Here's how the part is built. I have some questions about the finished solid (model axes, mm). A direction names the side the tool comes from. Round coordinates to 2 decimals unless told otherwise and drop trailing zeros. Write each loop counter-clockwise with the first axis right and the second up, starting at its lowest first coordinate (ties: lowest second). Pieces come first, ordered by that corner, then holes. Notation, with made-up numbers: (88, 68) - (132, 68) arc R16 cw to (132, 87) - close; hole circle Ø3 at (44, 27.5). An arc over 180 degrees is marked (long way). Use one line per item in the form item = value. Start each with the question number.
1. I want a section at A-A, the plane x = -13. List the corners of the cut face in (y, z) for me (3 decimals), plus the area to 3 significant figures.
2. Which directions (+Z, -Z, +X, -X, +Y, -Y) give clear straight access to the entire face, cutting with the end or side of a thin tool? Please do faces 1 (the flat face through (-21, 5, 17.805)), 2 (the flat face through (-99, 5, 14.805)), 3 (the flat face through (-86, 5, -86.155)).
3. I want a section at B-B, the plane y = 7. List the corners of the cut face in (x, z) for me (3 decimals), plus the area to 3 significant figures.
4. If I drill on line 1 along Z through (x, y) = (-58.5, 1) (3 decimals); line 2 along Z through (x, y) = (-132, 3.5) (3 decimals), over which ranges is the centre line in solid material (lowest first)?
5. Will these pins go through, and if not, where does the flat tip stop? pin 1 (2 mm diameter, centred on x = -5.5, y = 4, fed in from +Z) (3 decimals); pin 2 (1.8 mm diameter, centred on x = -52.5, y = 1, fed in from -Z) (3 decimals); pin 3 (3.5 mm diameter, centred on x = -6.49, z = 23.8, fed in from +Y); pin 4 (2.5 mm diameter, centred on x = -163.39, z = -91.16, fed in from -Y).
```python
from build123d import *

# Parameters (mm, degrees)
SKETCH1_R           = 1.5
BOSS_EXTRUDE1_DEPTH = 1.6
BOSS_EXTRUDE2_DEPTH = 7


with BuildPart() as part:
    # Sketch1 → Boss-Extrude1 (new body)
    with BuildSketch(Plane(origin=(0, 0, 0), x_dir=(1, 0, 0), z_dir=(0, 1, 0))):
        Polygon((-167.387715517, 87.155002586), (-167.387715517, -19.804997414), (-167.387715517, -28.459997414), (-159.387715517, -28.459997414), (-159.387715517, -19.804997414), (-10.487715517, -19.804997414), (-10.487715517, -28.459997414), (-2.487715517, -28.459997414), (-2.487715517, -19.804997414), (-2.487715517, 87.155002586), (-2.487715517, 95.810002586), (-10.487715517, 95.810002586), (-10.487715517, 87.155002586), (-159.387715517, 87.155002586), (-159.387715517, 95.810002586), (-167.387715517, 95.810002586), align=None)
        with Locations(Location((-6.487715517, -23.804997414, 0), (0, 0, 270))):
            Circle(SKETCH1_R, mode=Mode.SUBTRACT)
        with Locations(Location((-163.387715517, -23.804997414, 0), (0, 0, 270))):
            Circle(SKETCH1_R, mode=Mode.SUBTRACT)
        with Locations(Location((-6.487715517, 91.155002586, 0), (0, 0, 90))):
            Circle(SKETCH1_R, mode=Mode.SUBTRACT)
        with Locations(Location((-163.387715517, 91.155002586, 0), (0, 0, 90))):
            Circle(SKETCH1_R, mode=Mode.SUBTRACT)
    extrude(amount=BOSS_EXTRUDE1_DEPTH)

    # Sketch2 → Boss-Extrude2 (add)
    with BuildSketch(Plane(origin=(0, 1.6, 0), x_dir=(1, 0, 0), z_dir=(0, 1, 0))):
        Polygon((-167.387715517, 86.155002586), (-2.487715517, 86.155002586), (-2.487715517, -14.804997414), (-10.487715517, -14.804997414), (-10.487715517, -17.804997414), (-32.487715517, -17.804997414), (-32.487715517, -14.804997414), (-167.387715517, -14.804997414), align=None)
    extrude(amount=BOSS_EXTRUDE2_DEPTH)


solid = part.part
```
Model answer:
q1.outline = (0, -87.155) - (1.6, -87.155) - (1.6, -86.155) - (8.6, -86.155) - (8.6, 17.805) - (1.6, 17.805) - (1.6, 19.805) - (0, 19.805) - close
q1.area = 899 mm2
q2.face_1 = +Z, +X, -X, +Y
q2.face_2 = +Z, -X, +Y
q2.face_3 = -Z, +X, -X, +Y
q3.outline = (-167.388, -86.155) - (-2.488, -86.155) - (-2.488, 14.805) - (-10.488, 14.805) - (-10.488, 17.805) - (-32.488, 17.805) - (-32.488, 14.805) - (-167.388, 14.805) - close
q3.area = 16,700 mm2
q4.line_1 = -87.155 to 19.805
q4.line_2 = -86.155 to 14.805
q5.pin_1 = 14.805
q5.pin_2 = -87.155
q5.pin_3 = 1.6
q5.pin_4 = through
